from build123d import *

# Parameters (mm, degrees)
SKETCH_1_W          = 20
SKETCH_1_H          = 17.9
SKETCH_1_R          = 2.85
EXTRUDE_1_DEPTH     = 3
SKETCH_2_W          = 3
SKETCH_2_H          = 17.9
EXTRUDE_2_DEPTH     = 37
CUT_EXTRUDE_1_DEPTH = 37


with BuildPart() as part:
    # 草图1 → 凸台-拉伸1 (new body)
    with BuildSketch(Plane.XY):
        Rectangle(SKETCH_1_W, SKETCH_1_H)
        with Locations((0, -0.35)):
            Circle(SKETCH_1_R, mode=Mode.SUBTRACT)
    extrude(amount=EXTRUDE_1_DEPTH)

    # 草图2 → 凸台-拉伸2 (add)
    with BuildSketch(Plane.XY.offset(3)):
        with Locations((8.5, 0)):
            Rectangle(SKETCH_2_W, SKETCH_2_H)
    extrude(amount=EXTRUDE_2_DEPTH)

    # 草图3 → 切除-拉伸1 (cut)
    with BuildSketch(Plane.ZY.offset(-7)):
        with BuildLine():
            Line((32.15, -3.2), (9.65, -3.2))
            ThreePointArc((9.65, -3.2), (6.8, -0.35), (9.65, 2.5))
            Line((9.65, 2.5), (32.15, 2.5))
            ThreePointArc((32.15, 2.5), (35, -0.35), (32.15, -3.2))
        make_face()
    extrude(amount=-CUT_EXTRUDE_1_DEPTH, mode=Mode.SUBTRACT)


solid = part.part
Work out the finished part from the listing and answer in its coordinate system (mm). A direction names the side the tool comes from. Coordinates: 2 decimals unless noted, no trailing zeros. Write each loop counter-clockwise with the first axis right and the second up, starting at its lowest first coordinate (ties: lowest second). Pieces come first, ordered by that corner, then holes. Notation, with made-up numbers: M 17,31.25 L 71,31.25 A10 cw 71,45.25 Z; hole C 56.5,73 d3. An arc over 180 degrees is marked long. Write item = value, one per line.
1. For faces 1 (the face through (7.4, -8.95, 14)), 2 (the face through (8.5, -0.3, 35)), 3 (the face through (-4, 0, 3)), determine the directions among +Z, -Z, +X, -X, +Y, -Y from which every point of the face is accessible in a straight line to the end or side of a thin tool.
Solution:
face_1 = +Z, -Z, +X, -X, -Y
face_2 = +X, -X
face_3 = +Z, -X, +Y, -Y
2. The part is cut by section D-D (y = -0.35). Determine the outline of the cut face in (x, z), then the cut area to 3 significant figures.
Solution:
outline = M -10,0 L -2.85,0 L -2.85,3 L -10,3 Z; M 2.85,0 L 10,0 L 10,6.8 L 7,6.8 L 7,3 L 2.85,3 Z; M 7,35 L 10,35 L 10,40 L 7,40 Z
area = 69.3 mm2
3. Straight lines are drawn through the part: line 1 (Y direction, x = 0, z = 2.45); line 2 (Z direction, x = 3.5, y = 7.25); line 3 (X direction, y = -4, z = 11). For each, find the intervals that lie inside material, in ascending order. Write a range as from..to.
Solution:
line_1 = -8.95..-3.2, 2.5..8.95
line_2 = 0..3
line_3 = 7..10
4. Determine the mould class of faces 4 (the face through (7, 4, 21)), 5 (the face through (-2, 2, 0)), 6 (the face through (8, 2.5, 21)) for opening direction Z: released by +Z, released by -Z, zero draft, split by the parting line, or undercut.
Solution:
face_4 = zero draft
face_5 = released by -Z
face_6 = undercut
5. The part is cut by section B-B (z = 31.5). Determine the outline of the cut face in (x, y), then the cut area to 3 significant figures.
Solution:
outline = M 7,-8.95 L 10,-8.95 L 10,-3.2 L 7,-3.2 Z; M 7,2.5 L 10,2.5 L 10,8.95 L 7,8.95 Z
area = 36.6 mm2
6. The part is cut by section A-A (x = 0). Determine the outline of the cut face in (y, z).
Solution:
outline = M -8.95,0 L -3.2,0 L -3.2,3 L -8.95,3 Z; M 2.5,0 L 8.95,0 L 8.95,3 L 2.5,3 Z
7. The part is cut by section C-C (x = 8.5). Determine the outline of the cut face in (y, z), then the cut area to 3 significant figures.
Solution:
outline = M -8.95,0 L 8.95,0 L 8.95,40 L -8.95,40 Z; hole M -3.2,9.65 A2.85 ccw 2.5,9.65 L 2.5,32.15 A2.85 ccw -3.2,32.15 Z
area = 562 mm2
8. Flat-ended cylindrical pins translate along their axes: pin 1 (3 mm diameter, centred on y = -0.5, z = 35, fed in from -X); pin 2 (5 mm diameter, centred on x = 3, y = -4.5, fed in from +Z); pin 3 (4.5 mm diameter, centred on x = 0, y = -0.35, fed in from -Z). Find the tip coordinate at first contact, or state that the pin passes through.
Solution:
pin_1 = 7
pin_2 = 3
pin_3 = through
